from build123d import *

# Parameters (mm, degrees)
PAD_DEPTH       = 6
SKETCH001_R     = 2.75
PAD001_DEPTH    = 6
SKETCH002_R     = 2.75
POCKET_DEPTH    = 12.001
SKETCH003_R     = 6
SKETCH003_R_2   = 2.75
PAD002_DEPTH    = 5.3
SKETCH004_R     = 3.75
SKETCH004_R_2   = 2.75
PAD003_DEPTH    = 1
POCKET001_DEPTH = 9


with BuildPart() as part:
    # Sketch → Pad (new body)
    with BuildSketch(Plane.XY):
        Polygon((0, 0), (30, 0), (30, -15), (15, -30), (0, -30), align=None)
    extrude(amount=PAD_DEPTH)

    # Sketch001 (on Face6 of Pad) → Pad001 (join)
    with BuildSketch(Plane(origin=(0, 0, 0), x_dir=(1, 0, 0), z_dir=(0, 0, -1))):
        Polygon((15, 30), (-20, 30), (-20, 10), (0, 10), (0, 0), (10, 0), (10, -20), (30, -20), (30, 15), align=None)
        with Locations((-10, 20)):
            Circle(SKETCH001_R, mode=Mode.SUBTRACT)
        with Locations((20, -10)):
            Circle(SKETCH001_R, mode=Mode.SUBTRACT)
    extrude(amount=PAD001_DEPTH)

    # Sketch002 (on Face1 of Pad001) → Pocket (cut, through all)
    with BuildSketch(Plane.XY.offset(6)):
        with Locations((18, -18)):
            Circle(SKETCH002_R)
    extrude(amount=-POCKET_DEPTH, mode=Mode.SUBTRACT)

    # Sketch003 (on Face1 of Pocket) → Pad002 (join)
    with BuildSketch(Plane.XY.offset(6)):
        with Locations((18, -18)):
            Circle(SKETCH003_R)
        with Locations((18, -18)):
            Circle(SKETCH003_R_2, mode=Mode.SUBTRACT)
    extrude(amount=PAD002_DEPTH)

    # Sketch004 (on Face15 of Pad002) → Pad003 (join)
    with BuildSketch(Plane.XY.offset(11.3)):
        with Locations((18, -18)):
            Circle(SKETCH004_R)
        with Locations((18, -18)):
            Circle(SKETCH004_R_2, mode=Mode.SUBTRACT)
    extrude(amount=PAD003_DEPTH)

    # Sketch005 (on Face10 of Pad003) → Pocket001 (cut)
    with BuildSketch(Plane(origin=(0, 0, -6), x_dir=(1, 0, 0), z_dir=(0, 0, -1))):
        Polygon((22.75, 18), (20.375, 22.113621), (15.625, 22.113621), (13.25, 18), (15.625, 13.886379), (20.375, 13.886379), align=None)
    extrude(amount=-POCKET001_DEPTH, mode=Mode.SUBTRACT)


solid = part.part
Can you work these out from the model? Positions are in its coordinate system, mm. A direction names the side the tool comes from. Coordinates: 2 decimals unless noted, no trailing zeros. Order: outer loops, then holes, each group sorted by start corner. A loop starts at its lowest first (then second) coordinate and runs counter-clockwise, first axis right, second up. Notation, with made-up numbers: M 51,14.25 L 105,14.25 A20 ccw 105,18.25 Z; hole C 4,9.25 d8. An arc over 180 degrees is marked long. Write item = value, one per line.
(1) For pin 1 Ø3 at (x, z) = (-9, -2) entering from +Y; pin 2 Ø5 at (x, z) = (19, -3) entering from -Y; pin 3 Ø4 at (y, z) = (-8, 4) entering from -X, each with a flat end and sliding along its axis, tell me the tip position at first contact or that it passes through.
Results are:
pin_1 = -10
pin_2 = -28.5
pin_3 = 0
(2) I need wall thicknesses on line 1 along Y through (x, z) = (18, 12); line 2 along X through (y, z) = (10, -4.55); line 3 along Y through (x, z) = (-10, -3.7). Which ranges of each line are inside material? Lowest first, please. Write a range as [from, to].
Results are:
line_1 = [-21.75, -20.75], [-15.25, -14.25]
line_2 = [10, 17.25], [22.75, 30]
line_3 = [-30, -22.75], [-17.25, -10]
(3) Suppose I cut it at A-A on y = 10. Please give me the cut outline in (x, z).
Results are:
outline = M 10,-6 L 17.25,-6 L 17.25,0 L 10,0 Z; M 22.75,-6 L 30,-6 L 30,0 L 22.75,0 Z
(4) For faces 1 (the face through (21.58, -20.03, -1.56)), 2 (the face through (-10, -10, -3)), 3 (the face through (17.19, -21.66, 11.79)), 4 (the face through (17.253, 9.879, -2.958)), which set-ups out of +Z, -Z, +X, -X, +Y, -Y let a thin tool reach every point of the face, with its end or its side?
Results are:
face_1 = -Z
face_2 = +Z, -Z, -X, +Y
face_3 = +Z
face_4 = +Z, -Z
(5) Suppose I cut it at C-C on z = -2.5. Please give me the cut outline in (x, y) (3 decimals), plus the area to 3 significant figures.
Results are:
outline = M -20,-30 L 15,-30 L 30,-15 L 30,20 L 10,20 L 10,0 L 0,0 L 0,-10 L -20,-10 Z; hole C -10,-20 d5.5; hole M 13.25,-18 L 15.625,-22.114 L 20.375,-22.114 L 22.75,-18 L 20.375,-13.886 L 15.625,-13.886 Z; hole C 20,10 d5.5
area = 1,480 mm2
(6) Suppose I cut it at B-B on z = 1.5. Please give me the cut outline in (x, y) (3 decimals).
Results are:
outline = M 0,-30 L 15,-30 L 30,-15 L 30,0 L 0,0 Z; hole M 13.25,-18 L 15.625,-22.114 L 20.375,-22.114 L 22.75,-18 L 20.375,-13.886 L 15.625,-13.886 Z
(7) Suppose I cut it at D-D on y = -20. Please give me the cut outline in (x, z).
Results are:
outline = M -20,-6 L -12.75,-6 L -12.75,0 L -20,0 Z; M -7.25,-6 L 14.4,-6 L 14.4,3 L 16.11,3 L 16.11,12.3 L 14.83,12.3 L 14.83,11.3 L 12.34,11.3 L 12.34,6 L 0,6 L 0,0 L -7.25,0 Z; M 19.89,3 L 21.6,3 L 21.6,-6 L 25,-6 L 25,6 L 23.66,6 L 23.66,11.3 L 21.17,11.3 L 21.17,12.3 L 19.89,12.3 Z
